Read the model definition and answer for the solid it produces. Units are mm, in the model's axes. A direction names the side the tool comes from. Round coordinates to 2 decimals unless told otherwise and drop trailing zeros. Write each loop counter-clockwise with the first axis right and the second up, starting at its lowest first coordinate (ties: lowest second). Pieces come first, ordered by that corner, then holes. Notation, with made-up numbers: (2.5, 40) - (23.5, 40) arc R25 ccw to (23.5, 57) - close; hole circle Ø7 at (-15, 32.5). An arc over 180 degrees is marked (long way). One line per item, written item: value. Start each with the question number.
(1) Find the intervals of material crossed by L1, parallel to Y at x = -2.25, z = -3.5; L2, parallel to Y at x = -0.75, z = 1.75; L3, parallel to Z at x = 0.5, y = 23, in increasing order.
(2) The mould has two halves that part along X. Classify faces 1 (the face through (6, 7, 0)), 2 (the face through (0.05, 28.12, 1.48)), 3 (the face through (0, 23.6, -1.3)): +X half, -X half, draft (parallel to the pull), parting line (faces both ways), or undercut.
(3) A cutting plane is placed at A-A, the plane x = 0. Determine the outline of the cut face in (y, z) (3 decimals), plus the area to 3 significant figures.
(4) For faces 4 (the face through (-1.437, 23.22, -1.318)), 5 (the face through (5, 14, -4)), 6 (the face through (-5, 14, 4)), 7 (the face through (5, 14, 4)), determine the directions among +Z, -Z, +X, -X, +Y, -Y from which every point of the face is accessible in a straight line to the end or side of a thin tool.
(5) A cutting plane is placed at B-B, the plane z = 4.25. Determine the outline of the cut face in (x, y).
(6) A cutting plane is placed at D-D, the plane x = 5. Determine the outline of the cut face in (y, z) (3 decimals).
(7) Flat-ended cylindrical pins translate along their axes: pin 1 Ø1.5 at (x, z) = (-2.5, -4) entering from +Y; pin 2 Ø3 at (x, z) = (4.5, -2) entering from -Y; pin 3 Ø1.2 at (x, y) = (0, 26.5) entering from -Z. Find the tip coordinate at first contact, or state that the pin passes through.
(8) A cutting plane is placed at C-C, the plane y = 12.5. Determine the outline of the cut face in (x, z) (3 decimals), plus the area to 3 significant figures.
from build123d import *

# Parameters (mm, degrees)
BOSS_EXTRUDE1_DEPTH = 14
SKETCH3_W           = 12
SKETCH3_H           = 9.85
BOSS_EXTRUDE2_DEPTH = 8.85
SKETCH4_R           = 1.95
BOSS_EXTRUDE3_DEPTH = 0.75
BOSS_EXTRUDE4_DEPTH = 9.17
SKETCH6_R           = 2.47
BOSS_EXTRUDE5_DEPTH = 1.14


with BuildPart() as part:
    # Sketch2 → Boss-Extrude1 (new body)
    with BuildSketch(Plane(origin=(0, 0, 0), x_dir=(1, 0, 0), z_dir=(0, 1, 0))):
        with BuildLine():
            Line((-3.427006711, 4.925), (3.427006711, 4.925))
            ThreePointArc((3.427006711, 4.925), (6, 0), (3.427006711, -4.925))
            Line((3.427006711, -4.925), (-3.427006711, -4.925))
            ThreePointArc((-3.427006711, -4.925), (-6, 0), (-3.427006711, 4.925))
        make_face()
    extrude(amount=BOSS_EXTRUDE1_DEPTH)

    # Sketch3 → Boss-Extrude2 (add)
    with BuildSketch(Plane(origin=(0, 14, 0), x_dir=(1, 0, 0), z_dir=(0, 1, 0))):
        Rectangle(SKETCH3_W, SKETCH3_H)
    extrude(amount=BOSS_EXTRUDE2_DEPTH)

    # Sketch4 → Boss-Extrude3 (add)
    with BuildSketch(Plane(origin=(0, 22.85, 0), x_dir=(1, 0, 0), z_dir=(0, 1, 0))):
        Circle(SKETCH4_R)
    extrude(amount=BOSS_EXTRUDE3_DEPTH)

    # Sketch5 → Boss-Extrude4 (add)
    with BuildSketch(Plane(origin=(0, 23.6, 0), x_dir=(1, 0, 0), z_dir=(0, 1, 0))):
        with BuildLine():
            Line((-1.182497357, 0.89), (1.182497357, 0.89))
            ThreePointArc((1.182497357, 0.89), (0, -1.48), (-1.182497357, 0.89))
        make_face()
    extrude(amount=BOSS_EXTRUDE4_DEPTH)

    # Sketch6 → Boss-Extrude5 (add)
    with BuildSketch(Plane.XZ):
        Circle(SKETCH6_R)
    extrude(amount=BOSS_EXTRUDE5_DEPTH)


solid = part.part
Here are the results:
1. L1: 0 to 22.85
1. L2: -1.14 to 23.6
1. L3: -1.88 to 1.88
2. face 1: +X half
2. face 2: parting line
2. face 3: draft
3. outline: (-1.14, -2.47) - (0, -2.47) - (0, -4.925) - (22.85, -4.925) - (22.85, -1.95) - (23.6, -1.95) - (23.6, -0.89) - (32.77, -0.89) - (32.77, 1.48) - (23.6, 1.48) - (23.6, 1.95) - (22.85, 1.95) - (22.85, 4.925) - (0, 4.925) - (0, 2.47) - (-1.14, 2.47) - close
3. area: 255 mm²
4. face 4: +Y
4. face 5: -Z, +X, -Y
4. face 6: +Z, -X, -Y
4. face 7: +Z, +X, -Y
5. outline: (-6, 14) - (-4.24, 14) - (-4.24, 0) - (4.24, 0) - (4.24, 14) - (6, 14) - (6, 22.85) - (-6, 22.85) - close
6. outline: (0, -3.317) - (14, -3.317) - (14, -4.925) - (22.85, -4.925) - (22.85, 4.925) - (14, 4.925) - (14, 3.317) - (0, 3.317) - close
7. pin 1: y = 22.85
7. pin 2: y = 0
7. pin 3: z = -0.89
8. outline: (-3.427, -4.925) - (3.427, -4.925) arc R6 ccw to (3.427, 4.925) - (-3.427, 4.925) arc R6 ccw to start
8. area: 103 mm²
